The listing builds one solid part. Answer for the finished solid, in the listing's coordinates (mm). Give positions to 0.01 mm unless a question says otherwise; leave off trailing zeros. Order: outer loops, then holes, each group sorted by start corner. A loop starts at its lowest first (then second) coordinate and runs counter-clockwise, first axis right, second up. Notation, with made-up numbers: (0.25, 69.25) - (37.25, 69.25) arc R14 cw to (37.25, 96.25) - close; hole circle Ø7 at (71, 47). An arc over 180 degrees is marked (long way). Answer as a JSON object with one key per item and string values. Group by question number.
Q1. A cutting plane is placed at A-A, the plane z = 0. Give the vertices of the cut face in (x, y), and give its area (3 significant figures).
Q2. A cutting plane is placed at B-B, the plane y = 1. Give the vertices of the cut face in (x, z).
Q3. A cutting plane is placed at C-C, the plane z = 10.5. Give the vertices of the cut face in (x, y), and give its area (3 significant figures).
Q4. Consider line 1 (Z direction, x = -127, y = -0.2); line 2 (X direction, y = -1.95, z = 4); line 3 (X direction, y = 0.85, z = -11). Determine where each line is inside the solid, lowest interval first.
Q5. The mould has two halves that part along X. Classify faces 1 (the face through (-8, -2.381, 0)), 2 (the face through (-139.697, -0.033, 0.279)), 3 (the face through (127, 0, 0)), 4 (the face through (-120.943, 0.033, 1.907)): released by +X, released by -X, zero draft, split by the parting line, or undercut.
from build123d import *

# Parameters (mm, degrees)
F0_R     = 6.35
F1_DEPTH = 2.38125


with BuildPart() as f1:
    # F0 (on Front) → F1 (new body, symmetric)
    with BuildSketch(Plane.XZ):
        with BuildLine():
            ThreePointArc((-127, 12.7), (-139.7, 0), (-127, -12.7))
            Line((-127, -12.7), (127, -12.7))
            Line((127, -12.7), (127, 12.7))
            Line((127, 12.7), (-127, 12.7))
        make_face()
        with Locations((-127, 0)):
            Circle(F0_R, mode=Mode.SUBTRACT)
    extrude(amount=F1_DEPTH, both=True)


solid = f1.part
Reply:
{
 "1": {"outline": "(-139.7, -2.38) - (-133.35, -2.38) - (-133.35, 2.38) - (-139.7, 2.38) - close; (-120.65, -2.38) - (127, -2.38) - (127, 2.38) - (-120.65, 2.38) - close", "area": "1,210 mm^2"},
 "2": {"outline": "(-127, -12.7) - (127, -12.7) - (127, 12.7) - (-127, 12.7) arc R12.7 ccw to start; hole circle Ø12.7 at (-127, 0)"},
 "3": {"outline": "(-134.14, -2.38) - (127, -2.38) - (127, 2.38) - (-134.14, 2.38) - close", "area": "1,240 mm^2"},
 "4": {"line 1": "z = -12.7 to -6.35, 6.35 to 12.7", "line 2": "x = -139.05 to -131.93, -122.07 to 127", "line 3": "x = -133.35 to 127"},
 "5": {"face 1": "zero draft", "face 2": "released by -X", "face 3": "released by +X", "face 4": "undercut"}
}
